```python
from build123d import *

# Parameters (mm, degrees)
SKETCH10_R              = 4.7625
CUT_EXTRUDE4_DEPTH      = 11.31875
CUT_EXTRUDE4_DEPTH_BACK = 11.31875
SKETCH12_R              = 6.6675
SKETCH12_R_2            = 4.7625
EXTRUDE1_DEPTH          = 11.1125
EXTRUDE1_DEPTH_BACK     = 11.1125
CHAMFER1_SIZE           = 0.47625


with BuildPart() as part:
    # Sketch7 → Revolve3 (revolve)
    with BuildSketch(Plane.XY):
        with BuildLine():
            Line((0, 29.36875), (0, 8.73125))
            ThreePointArc((0, 8.73125), (10.31875, 19.05), (0, 29.36875))
        make_face()
    revolve(axis=Axis((0, 0, 0), (0, 1, 0)))

    # Sketch10 → Cut-Extrude4 (cut, two sides)
    with BuildSketch(Plane.XY) as cut_extrude4_sk:
        with Locations((0, 19.05)):
            Circle(SKETCH10_R)
    extrude(amount=CUT_EXTRUDE4_DEPTH, mode=Mode.SUBTRACT)
    extrude(cut_extrude4_sk.sketch, amount=-CUT_EXTRUDE4_DEPTH_BACK, mode=Mode.SUBTRACT)

    # Sketch12 → Extrude1 (add, two sides)
    with BuildSketch(Plane.XY) as extrude1_sk:
        with Locations((0, 19.05)):
            Circle(SKETCH12_R)
        with Locations((0, 19.05)):
            Circle(SKETCH12_R_2, mode=Mode.SUBTRACT)
    extrude(amount=EXTRUDE1_DEPTH)
    extrude(extrude1_sk.sketch, amount=-EXTRUDE1_DEPTH_BACK)

    # Chamfer1
    chamfer1_edges = [part.edges().sort_by_distance(p)[0] for p in [
        (-4.7625, 19.05, 11.1125),
        (-4.7625, 19.05, -11.1125),
    ]]
    chamfer(chamfer1_edges, length=CHAMFER1_SIZE)


solid = part.part
```
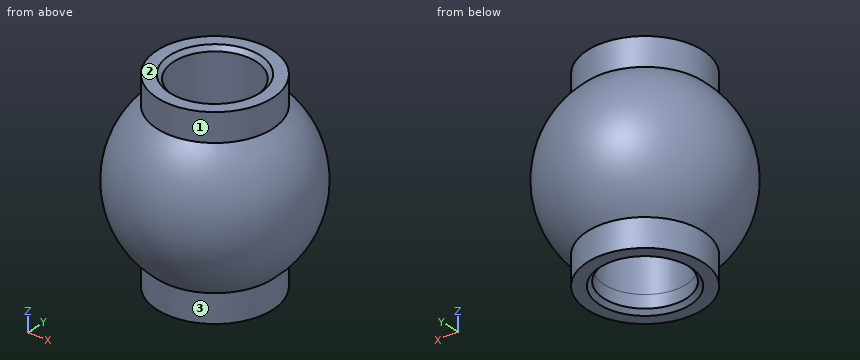
Here's how the part is built. I have some questions about the finished solid (model axes, mm). Face numbers are marked on the shaded views. A direction names the side the tool comes from. Give positions to 0.01 mm unless a question says otherwise; leave off trailing zeros. Order: outer loops, then holes, each group sorted by start corner. A loop starts at its lowest first (then second) coordinate and runs counter-clockwise, first axis right, second up. Notation, with made-up numbers: (-24, 31.5) - (-14, 31.5) arc R26 ccw to (-14, 47.5) - close; hole circle Ø2 at (72.5, -31.75). An arc over 180 degrees is marked (long way). Answer as a JSON object with one key per item and string values. Group by question number.
Item 1: If we section it at D-D on y = 13.25: Please give me the cut outline in (x, z), and give its area (3 significant figures).
Item 2: If we section it at A-A on y = 19.05: Please give me the cut outline in (x, z).
Item 3: Please list where these lines run through material, in increasing order: probe 1 along Y at (x, z) = (0, -9.6); probe 2 along Y at (x, z) = (0, 0.25); probe 3 along X at (y, z) = (19.05, -10).
Item 4: Which directions (+Z, -Z, +X, -X, +Y, -Y) give clear straight access to the entire face, cutting with the end or side of a thin tool? Please do the marked faces 1, 2 and 3.
Item 5: If we section it at B-B on x = 0: Please give me the cut outline in (y, z), and give its area (3 significant figures).
Item 6: For P1, Ø12, axis at y = 13.5, z = -6, coming from the +X side; P2, Ø10, axis at x = 1.5, z = -4, coming from the -Y side; P3, Ø1.5, axis at y = 17, z = -5, coming from the -X side; P4, Ø10, axis at x = 0.5, z = -6, coming from the +Y side, each with a flat end and sliding along its axis, tell me the tip position at first contact or that it passes through.
Result set:
{
 "1": {"outline": "(-3.29, -11.11) - (3.29, -11.11) - (3.29, -7.88) arc R8.53 ccw to (3.29, 7.88) - (3.29, 11.11) - (-3.29, 11.11) - (-3.29, 7.88) arc R8.53 ccw to (-3.29, -7.88) - close", "area": "266 mm²"},
 "2": {"outline": "(-6.67, -11.11) - (-5.24, -11.11) - (-4.76, -10.64) - (-4.76, 10.64) - (-5.24, 11.11) - (-6.67, 11.11) - (-6.67, 7.88) arc R10.32 ccw to (-6.67, -7.88) - close; (4.76, -10.64) - (5.24, -11.11) - (6.67, -11.11) - (6.67, -7.88) arc R10.32 ccw to (6.67, 7.88) - (6.67, 11.11) - (5.24, 11.11) - (4.76, 10.64) - close"},
 "3": {"probe 1": "12.38 to 14.29, 23.81 to 25.72", "probe 2": "8.73 to 14.29, 23.81 to 29.37", "probe 3": "-6.67 to -4.76, 4.76 to 6.67"},
 "4": {"face 1": "+Z", "face 2": "+Z, +X, -X, +Y, -Y", "face 3": "-Z"},
 "5": {"outline": "(12.38, -11.11) - (13.81, -11.11) - (14.29, -10.64) - (14.29, 10.64) - (13.81, 11.11) - (12.38, 11.11) - (12.38, 7.88) arc R10.32 ccw to (12.38, -7.88) - close; (23.81, -10.64) - (24.29, -11.11) - (25.72, -11.11) - (25.72, -7.88) arc R10.32 ccw to (25.72, 7.88) - (25.72, 11.11) - (24.29, 11.11) - (23.81, 10.64) - close", "area": "164 mm²"},
 "6": {"P1": "x = 10.09", "P2": "y = 8.73", "P3": "x = -9.21", "P4": "y = 29.32"}
}
